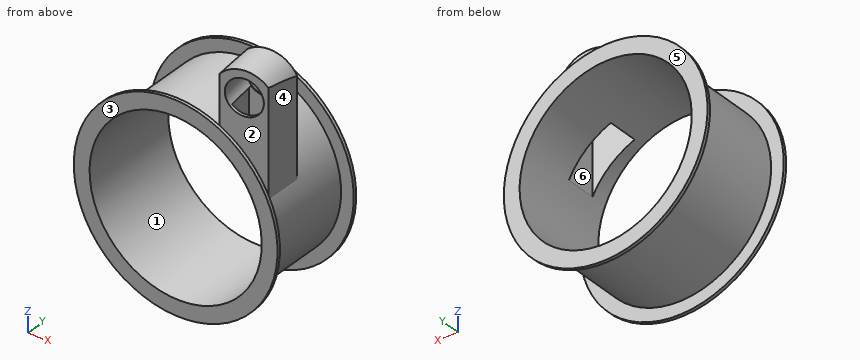
```python
from build123d import *

# Parameters (mm, degrees)
BOSS_EXTRUDE2_DEPTH     = 101
CUT_EXTRUDE3_DEPTH      = 427.519947779
CUT_EXTRUDE3_DEPTH_BACK = 427.519947779
CUT_EXTRUDE4_DEPTH      = 424.573467382
CUT_EXTRUDE4_DEPTH_BACK = 64
SKETCH5_R               = 28.146504222
CUT_EXTRUDE7_DEPTH      = 36
CUT_EXTRUDE7_DEPTH_BACK = 113
CUT_EXTRUDE8_DEPTH      = 414.870820929
CUT_EXTRUDE8_DEPTH_BACK = 414.870820929
SKETCH8_R               = 136.4


with BuildPart() as part:
    # Sketch1 → Revolve1 (revolve)
    with BuildSketch(Plane.XY, mode=Mode.PRIVATE) as revolve1_sk:
        Polygon((0, 0), (-20, 0), (-20, -5), (5, -5), (141.4, -5), (141.4, 150), (141.4, 155), (-20, 155), (-20, 150), (0, 150), align=None)
    revolve(revolve1_sk.sketch.rotate(Axis((141.4, 150, 0), (0, -1, 0)), 270), axis=Axis((141.4, 150, 0), (0, -1, 0)))

    # Sketch3 → Boss-Extrude2 (add, symmetric)
    with BuildSketch(Plane.XY.offset(140)):
        Polygon((271.787755102, 74.631332533), (201.787755102, 64.685114046), (201.787755102, 6.428691477), (271.787755102, 16.374909964), align=None)
    extrude(amount=BOSS_EXTRUDE2_DEPTH, both=True)

    # Sketch4 → Cut-Extrude3 (cut, two sides: drawn at the far end of the back side and taken through both)
    with BuildSketch(Plane(origin=(4.504708933, -31.703468583, 0), x_dir=(-0.9900557063765247, -0.1406758624330439, 0), z_dir=(0.1406758624330439, -0.9900557063765248, 0)).offset(-CUT_EXTRUDE3_DEPTH_BACK)):
        with BuildLine():
            Line((-283.0966697, -198.98279485), (-292.524457183, -243.549272165))
            Line((-292.524457183, -243.549272165), (-246.6966359, -274.042125065))
            Line((-246.6966359, -274.042125065), (-190.71002304, -274.042125065))
            Line((-190.71002304, -274.042125065), (-190.71002304, -198.98279485))
            ThreePointArc((-190.71002304, -198.98279485), (-236.90334637, -235.746084626), (-283.0966697, -198.98279485))
        make_face()
    extrude(amount=CUT_EXTRUDE3_DEPTH + CUT_EXTRUDE3_DEPTH_BACK, mode=Mode.SUBTRACT)

    # Sketch5 → Cut-Extrude4 (cut, two sides: drawn at the far end of the back side and taken through both)
    with BuildSketch(Plane(origin=(4.504708933, -31.703468583, 0), x_dir=(-0.9900557063765247, -0.1406758624330439, 0), z_dir=(0.1406758624330439, -0.9900557063765248, 0)).offset(-CUT_EXTRUDE4_DEPTH_BACK)):
        with Locations((-236.587007924, -195.244994695)):
            Circle(SKETCH5_R)
    extrude(amount=CUT_EXTRUDE4_DEPTH + CUT_EXTRUDE4_DEPTH_BACK, mode=Mode.SUBTRACT)

    # Sketch6 → Cut-Extrude7 (cut, two sides: drawn at the far end of the back side and taken through both)
    with BuildSketch(Plane.XY.offset(140).offset(-CUT_EXTRUDE7_DEPTH_BACK)):
        Polygon((206.787755102, 60.42244898), (206.787755102, 12.189356534), (266.787755102, 20.714686666), (266.787755102, 68.852201046), align=None)
    extrude(amount=CUT_EXTRUDE7_DEPTH + CUT_EXTRUDE7_DEPTH_BACK, mode=Mode.SUBTRACT)

    # Sketch8 → Cut-Extrude8 (cut, two sides: drawn at the far end of the back side and taken through both)
    with BuildSketch(Plane(origin=(0, 0, 0), x_dir=(1, 0, 0), z_dir=(0, 1, 0)).offset(-CUT_EXTRUDE8_DEPTH_BACK)):
        with Locations(Location((141.4, 0, 0), (0, 0, 270))):
            Circle(SKETCH8_R)
    extrude(amount=CUT_EXTRUDE8_DEPTH + CUT_EXTRUDE8_DEPTH_BACK, mode=Mode.SUBTRACT)


solid = part.part
```
Input: part model. Units: mm. Frame: model coordinates. Face numbers are marked on the shaded views. A direction names the side the tool comes from. Give positions to 0.01 mm unless a question says otherwise; leave off trailing zeros. Loops run counter-clockwise (first coordinate to the right, second up) from the corner with the lowest first, then second, coordinate; pieces in that order, holes last. Notation, with made-up numbers: M 84,-37.75 L 106,-37.75 A10 cw 106,-26.75 Z; hole C 40.5,63.5 d2. An arc over 180 degrees is marked long. Answer as CSV lines item,"result". Start each with the question number.
1. Pin query (flat end, axial travel): P1, Ø8, axis at x = 253.5, z = 186.5, coming from the +Y side; P2, Ø14.5, axis at y = 48.5, z = 100, coming from the -X side; P3, Ø10.5, axis at x = 211, y = 31, coming from the -Z side. Return the tip coordinate at first contact, or that it passes through.
2. Pull-direction query (X, two-part tool) for the marked faces 1, 2 and 3; classes: released by +X, released by -X, zero draft, split by the parting line, or undercut.
3. Section A-A on x = 141.4. Return loops of the section in (y, z).
4. Line query: L1, parallel to X at y = 75, z = 0; L2, parallel to Y at x = 44.5, z = 104.5; L3, parallel to Z at x = 141, y = 41. Output: solid intervals per line, ascending.
5. Section B-B on z = -121.5. Return loops of the section in (x, y), plus the area to 3 significant figures.
6. Reachability of the marked faces 4, 5 and 6 from +Z, -Z, +X, -X, +Y, -Y: full face, straight path, thin tool, end or side. Return the list, or none.
7. Section C-C on y = 87.5. Return loops of the section in (x, z).
Computed values:
1,P1,"stops at y = 72.6"
1,P2,"stops at x = 34.67"
1,P3,"stops at z = -125.91"
2,face 1,"undercut"
2,face 2,"released by +X"
2,face 3,"zero draft"
3,outline,"M -5,-161.4 L 0,-161.4 L 0,-141.4 L 150,-141.4 L 150,-161.4 L 155,-161.4 L 155,-136.4 L -5,-136.4 Z; M -5,136.4 L 155,136.4 L 155,161.4 L 150,161.4 L 150,141.4 L 0,141.4 L 0,161.4 L -5,161.4 Z"
4,L1,"x = 0 to 5, 277.8 to 282.8"
4,L2,"y = -5 to 0, 150 to 155"
4,L3,"z = -141.4 to -136.4, 136.4 to 141.4"
5,outline,"M 35.16,-5 L 79.41,-5 L 79.41,155 L 35.16,155 L 35.16,150 L 69.07,150 L 69.07,0 L 35.16,0 Z; M 203.39,-5 L 247.64,-5 L 247.64,0 L 213.73,0 L 213.73,150 L 247.64,150 L 247.64,155 L 203.39,155 Z"
5,area,"3,990 mm²"
6,face 4,"+Z, +X"
6,face 5,"+Z, -Z, +X, -X, +Y"
6,face 6,"none"
7,outline,"C 141.4,0 d282.8; hole C 141.4,0 d272.8"
